Geometry check sheet. Reference: the model listing, model coordinates, mm. Face numbers are marked on the shaded views. A direction names the side the tool comes from. Coordinates: 2 decimals unless noted, no trailing zeros. Loops run counter-clockwise (first coordinate to the right, second up) from the corner with the lowest first, then second, coordinate; pieces in that order, holes last. Notation, with made-up numbers: M 73.5,6 L 131.5,6 A17 ccw 131.5,21 Z; hole C 23,25.5 d5. An arc over 180 degrees is marked long. One line per question, with ' | ' between items. Start each with the question number.
from build123d import *

# Parameters (mm, degrees)
SKETCH1_W                      = 100
SKETCH1_H                      = 59
BOSS_EXTRUDE1_DEPTH            = 12
SKETCH2_W                      = 92
SKETCH2_H                      = 54
CUT_EXTRUDE1_DEPTH             = 60.281109976
SKETCH3_W                      = 54
SKETCH3_H                      = 2.75
CUT_EXTRUDE2_DEPTH             = 1.25
SKETCH4_W                      = 54
SKETCH4_H                      = 2.75
CUT_EXTRUDE3_DEPTH             = 1.25
SKETCH5_W                      = 92
SKETCH5_H                      = 2.75
CUT_EXTRUDE4_DEPTH             = 1.25
SKETCH6_W                      = 92
SKETCH6_H                      = 2.75
CUT_EXTRUDE5_DEPTH             = 1.25
FILLET1_R                      = 1
SKETCH7_W                      = 4
SKETCH7_H                      = 10
BOSS_EXTRUDE2_DEPTH            = 5
CUT_EXTRUDE6_REACH             = 103.145
SKETCH8_W                      = 8
SKETCH8_H                      = 3
CUT_EXTRUDE6_DIRECTION_2_REACH = 103.145
FILLET2_R                      = 6.35
SKETCH9_W                      = 5
SKETCH9_H                      = 2.5
BOSS_EXTRUDE3_DEPTH            = 5
SKETCH10_W                     = 5
SKETCH10_H                     = 2.5
BOSS_EXTRUDE4_DEPTH            = 5
SKETCH11_W                     = 5
SKETCH11_H                     = 2.5
BOSS_EXTRUDE5_DEPTH            = 5
SKETCH12_W                     = 5
SKETCH12_H                     = 2.5
BOSS_EXTRUDE6_DEPTH            = 4


with BuildPart() as part:
    # Sketch1 → Boss-Extrude1 (new body)
    with BuildSketch(Plane(origin=(0, 0, 0), x_dir=(1, 0, 0), z_dir=(0, 1, 0))):
        Rectangle(SKETCH1_W, SKETCH1_H)
    extrude(amount=BOSS_EXTRUDE1_DEPTH)

    # Sketch2 → Cut-Extrude1 (cut, through all)
    with BuildSketch(Plane(origin=(0, 12, 0), x_dir=(1, 0, 0), z_dir=(0, 1, 0))):
        Rectangle(SKETCH2_W, SKETCH2_H)
    extrude(amount=-CUT_EXTRUDE1_DEPTH, mode=Mode.SUBTRACT)

    # Sketch3 → Cut-Extrude2 (cut)
    with BuildSketch(Plane(origin=(-46, 0, 0), x_dir=(0, 0, -1), z_dir=(1, 0, 0))):
        with Locations((0, 3.875)):
            Rectangle(SKETCH3_W, SKETCH3_H)
    extrude(amount=-CUT_EXTRUDE2_DEPTH, mode=Mode.SUBTRACT)

    # Sketch4 → Cut-Extrude3 (cut)
    with BuildSketch(Plane.ZY.offset(-46)):
        with Locations((0, 3.875)):
            Rectangle(SKETCH4_W, SKETCH4_H)
    extrude(amount=-CUT_EXTRUDE3_DEPTH, mode=Mode.SUBTRACT)

    # Sketch5 → Cut-Extrude4 (cut)
    with BuildSketch(Plane.XY.offset(-27)):
        with Locations((0, 3.875)):
            Rectangle(SKETCH5_W, SKETCH5_H)
    extrude(amount=-CUT_EXTRUDE4_DEPTH, mode=Mode.SUBTRACT)

    # Sketch6 → Cut-Extrude5 (cut)
    with BuildSketch(Plane(origin=(0, 0, 27), x_dir=(-1, 0, 0), z_dir=(0, 0, -1))):
        with Locations((0, 3.875)):
            Rectangle(SKETCH6_W, SKETCH6_H)
    extrude(amount=-CUT_EXTRUDE5_DEPTH, mode=Mode.SUBTRACT)

    # Fillet1
    fillet1_edges = [part.edges().sort_by_distance(p)[0] for p in [
        (0, 5.25, -28.25),
        (0, 5.25, 28.25),
    ]]
    fillet(fillet1_edges, radius=FILLET1_R)

    # Sketch7 → Boss-Extrude2 (add)
    with BuildSketch(Plane.XZ):
        with Locations((-48, 0)):
            Rectangle(SKETCH7_W, SKETCH7_H)
    boss_extrude2 = extrude(amount=BOSS_EXTRUDE2_DEPTH)

    # Mirror2: Boss-Extrude2 across plane
    add(boss_extrude2.mirror(Plane(origin=(0, 0, 0), x_dir=(0, 0, 1), z_dir=(1, 0, 0))))

    # Cut-Extrude6: up to this face of the body (flat: up to its plane)
    cut_extrude6_end = Plane(part.part.faces().sort_by_distance((-47.25, 3.875, 0))[0])
    # Sketch8 → Cut-Extrude6 (cut, up to the picked face)
    with BuildSketch(Plane(origin=(-46, 0, 0), x_dir=(0, 0, -1), z_dir=(1, 0, 0)), mode=Mode.PRIVATE) as cut_extrude6_sk1:
        with Locations((0, 1)):
            Rectangle(SKETCH8_W, SKETCH8_H)
    cut_extrude6_tool1 = split(extrude(cut_extrude6_sk1.sketch, amount=-CUT_EXTRUDE6_REACH, mode=Mode.PRIVATE), bisect_by=cut_extrude6_end, keep=Keep.BOTH, mode=Mode.PRIVATE)
    add(cut_extrude6_tool1.solids().sort_by(Axis((-46, 1, 0), (-1, 0, 0)))[0], mode=Mode.SUBTRACT)

    # Cut-Extrude6 direction 2: up to this face of the body (flat: up to its plane)
    cut_extrude6_direction_2_end = Plane(part.part.faces().sort_by_distance((47.25, 3.875, 0))[0])
    # Sketch8 → Cut-Extrude6 direction 2 (cut, up to the picked face)
    with BuildSketch(Plane(origin=(-46, 0, 0), x_dir=(0, 0, -1), z_dir=(1, 0, 0)), mode=Mode.PRIVATE) as cut_extrude6_direction_2_sk1:
        with Locations((0, 1)):
            Rectangle(SKETCH8_W, SKETCH8_H)
    cut_extrude6_direction_2_tool1 = split(extrude(cut_extrude6_direction_2_sk1.sketch, amount=CUT_EXTRUDE6_DIRECTION_2_REACH, mode=Mode.PRIVATE), bisect_by=cut_extrude6_direction_2_end, keep=Keep.BOTH, mode=Mode.PRIVATE)
    add(cut_extrude6_direction_2_tool1.solids().sort_by(Axis((-46, 1, 0), (1, 0, 0)))[0], mode=Mode.SUBTRACT)

    # Fillet2
    # the kernel refuses this fillet: 6.35 mm, written as the material it adds along each edge
    with BuildSketch(Plane(origin=(-46, 18.375, -27), x_dir=(1, 0, 0), z_dir=(0, -1, 0))) as fillet2_piece_1_section:
        with BuildLine():
            CenterArc((FILLET2_R, FILLET2_R), FILLET2_R, 180, 90)
            Line((0, FILLET2_R), (0, 0))
            Line((0, 0), (FILLET2_R, 0))
        make_face()
    fillet2_piece_1 = extrude(amount=18.375, mode=Mode.PRIVATE)
    fillet2_piece_1 = split(fillet2_piece_1, bisect_by=Plane(origin=(-44.562391024, 5.25, -25.562391024), z_dir=(0, 1, 0)), keep=Keep.TOP, mode=Mode.PRIVATE)
    fillet2_piece_1 = split(fillet2_piece_1, bisect_by=Plane(origin=(-44.562391024, 12, -25.562391024), z_dir=(0, -1, 0)), keep=Keep.TOP, mode=Mode.PRIVATE)
    add(fillet2_piece_1)
    with BuildSketch(Plane(origin=(-46, 2.5, -27), x_dir=(1, 0, 0), z_dir=(0, -1, 0)), Plane(origin=(-46, 2.5, 27), x_dir=(0, 0, -1), z_dir=(0, -1, 0))) as fillet2_piece_2:
        with BuildLine():
            CenterArc((FILLET2_R, FILLET2_R), FILLET2_R, 180, 90)
            Line((0, FILLET2_R), (0, 0))
            Line((0, 0), (FILLET2_R, 0))
        make_face()
    extrude(amount=2.5)
    with BuildSketch(Plane(origin=(46, 18.375, -27), x_dir=(-1, 0, 0), z_dir=(0, -1, 0))) as fillet2_piece_3_section:
        with BuildLine():
            CenterArc((FILLET2_R, -FILLET2_R), FILLET2_R, 90, 90)
            Line((0, -FILLET2_R), (0, 0))
            Line((0, 0), (FILLET2_R, 0))
        make_face()
    fillet2_piece_3 = extrude(amount=18.375, mode=Mode.PRIVATE)
    fillet2_piece_3 = split(fillet2_piece_3, bisect_by=Plane(origin=(44.562391024, 5.25, -25.562391024), z_dir=(0, 1, 0)), keep=Keep.TOP, mode=Mode.PRIVATE)
    fillet2_piece_3 = split(fillet2_piece_3, bisect_by=Plane(origin=(44.562391024, 12, -25.562391024), z_dir=(0, -1, 0)), keep=Keep.TOP, mode=Mode.PRIVATE)
    add(fillet2_piece_3)
    with BuildSketch(Plane(origin=(46, 2.5, -27), x_dir=(-1, 0, 0), z_dir=(0, -1, 0)), Plane(origin=(46, 2.5, 27), x_dir=(0, 0, -1), z_dir=(0, -1, 0))) as fillet2_piece_4:
        with BuildLine():
            CenterArc((FILLET2_R, -FILLET2_R), FILLET2_R, 90, 90)
            Line((0, -FILLET2_R), (0, 0))
            Line((0, 0), (FILLET2_R, 0))
        make_face()
    extrude(amount=2.5)
    with BuildSketch(Plane(origin=(-46, 18.375, 27), x_dir=(0, 0, -1), z_dir=(0, -1, 0))) as fillet2_piece_5_section:
        with BuildLine():
            CenterArc((FILLET2_R, FILLET2_R), FILLET2_R, 180, 90)
            Line((0, FILLET2_R), (0, 0))
            Line((0, 0), (FILLET2_R, 0))
        make_face()
    fillet2_piece_5 = extrude(amount=18.375, mode=Mode.PRIVATE)
    fillet2_piece_5 = split(fillet2_piece_5, bisect_by=Plane(origin=(-44.562391024, 12, 25.562391024), z_dir=(0, -1, 0)), keep=Keep.TOP, mode=Mode.PRIVATE)
    fillet2_piece_5 = split(fillet2_piece_5, bisect_by=Plane(origin=(-44.562391024, 5.25, 25.562391024), z_dir=(0, 1, 0)), keep=Keep.TOP, mode=Mode.PRIVATE)
    add(fillet2_piece_5)
    with BuildSketch(Plane(origin=(46, 18.375, 27), x_dir=(0, 0, -1), z_dir=(0, -1, 0))) as fillet2_piece_6_section:
        with BuildLine():
            CenterArc((FILLET2_R, -FILLET2_R), FILLET2_R, 90, 90)
            Line((0, -FILLET2_R), (0, 0))
            Line((0, 0), (FILLET2_R, 0))
        make_face()
    fillet2_piece_6 = extrude(amount=18.375, mode=Mode.PRIVATE)
    fillet2_piece_6 = split(fillet2_piece_6, bisect_by=Plane(origin=(44.562391024, 12, 25.562391024), z_dir=(0, -1, 0)), keep=Keep.TOP, mode=Mode.PRIVATE)
    fillet2_piece_6 = split(fillet2_piece_6, bisect_by=Plane(origin=(44.562391024, 5.25, 25.562391024), z_dir=(0, 1, 0)), keep=Keep.TOP, mode=Mode.PRIVATE)
    add(fillet2_piece_6)
    # the kernel refuses this fillet: 6.35 mm, written as the material it takes off along each edge
    with BuildSketch(Plane(origin=(-50, -15.875, -29.5), x_dir=(1, 0, 0), z_dir=(0, 1, 0)), Plane(origin=(-50, -15.875, 29.5), x_dir=(0, 0, -1), z_dir=(0, 1, 0))) as fillet2_2_piece_1:
        with BuildLine():
            CenterArc((FILLET2_R, -FILLET2_R), FILLET2_R, 90, 90)
            Line((0, -FILLET2_R), (0, 0))
            Line((0, 0), (FILLET2_R, 0))
        make_face()
    extrude(amount=43.75, mode=Mode.SUBTRACT)
    with BuildSketch(Plane(origin=(50, -15.875, 29.5), x_dir=(0, 0, -1), z_dir=(0, 1, 0)), Plane(origin=(50, -15.875, -29.5), x_dir=(-1, 0, 0), z_dir=(0, 1, 0))) as fillet2_2_piece_2:
        with BuildLine():
            CenterArc((FILLET2_R, FILLET2_R), FILLET2_R, 180, 90)
            Line((0, FILLET2_R), (0, 0))
            Line((0, 0), (FILLET2_R, 0))
        make_face()
    extrude(amount=43.75, mode=Mode.SUBTRACT)

    # Sketch9 → Boss-Extrude3 (add)
    with BuildSketch(Plane(origin=(0, 0, 27), x_dir=(-1, 0, 0), z_dir=(0, 0, -1))):
        with Locations((0, 7.5)):
            Rectangle(SKETCH9_W, SKETCH9_H)
    extrude(amount=BOSS_EXTRUDE3_DEPTH)

    # Sketch10 → Boss-Extrude4 (add)
    with BuildSketch(Plane.XY.offset(-27)):
        with Locations((0, 7.5)):
            Rectangle(SKETCH10_W, SKETCH10_H)
    extrude(amount=BOSS_EXTRUDE4_DEPTH)

    # Sketch11 → Boss-Extrude5 (add)
    with BuildSketch(Plane.ZY.offset(-46)):
        with Locations((0, 7.5)):
            Rectangle(SKETCH11_W, SKETCH11_H)
    extrude(amount=BOSS_EXTRUDE5_DEPTH)

    # Sketch12 → Boss-Extrude6 (add)
    with BuildSketch(Plane(origin=(-46, 0, 0), x_dir=(0, 0, -1), z_dir=(1, 0, 0))):
        with Locations((0, 7.5)):
            Rectangle(SKETCH12_W, SKETCH12_H)
    extrude(amount=BOSS_EXTRUDE6_DEPTH)


solid = part.part
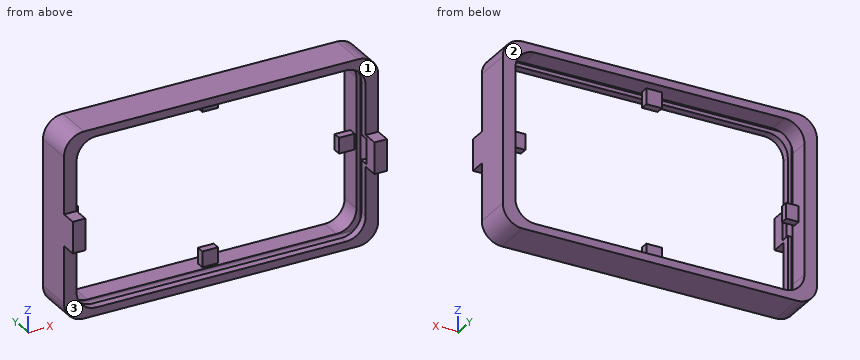
1. Sectioned sample at C-C (z = 13.5). Record the cut outline in (x, y).
2. Depth check by flat-ended pin: pin 1 Ø0.6 at (y, z) = (4, -27.5) entering from -X; pin 2 Ø1.4 at (y, z) = (4.5, 27.5) entering from -X; pin 3 Ø2 at (y, z) = (7.5, 24.5) entering from +X. Enter the tip coordinate at first touch or a pass-through.
3. Thickness scan on line 1 (X direction, y = 3.25, z = -12.5); line 2 (X direction, y = 7.5, z = -18.5); line 3 (Z direction, x = -17.5, y = 4.25). Record the ranges inside material, lowest first.
4. Tool access check on the marked faces 1, 2 and 3. Record the directions out of +Z, -Z, +X, -X, +Y, -Y that give a thin tool (end or side, any length) a straight path to the whole face; none if there is none.
5. Sectioned sample at A-A (x = -32). Record the cut outline in (y, z), and give its area (3 significant figures).
6. Sectioned sample at D-D (y = -3). Record the cut outline in (x, z).
Result:
1) outline: M -50,0 L -46,0 L -46,2.5 L -47.25,2.5 L -47.25,5.25 L -46,5.25 L -46,12 L -50,12 Z; M 46,0 L 50,0 L 50,12 L 46,12 L 46,5.25 L 47.25,5.25 L 47.25,2.5 L 46,2.5 Z
2) pin 1: stops at x = -48.54 | pin 2: stops at x = -48.85 | pin 3: stops at x = 49.99
3) line 1: x = -50 to -47.25, 47.25 to 50 | line 2: x = -50 to -46, 46 to 50 | line 3: z = -29.5 to -28.25, 28.25 to 29.5
4) face 1: +Z, +X, -X, -Y | face 2: +Z, -Z, +X, -X, +Y | face 3: -Z, +X, -X, -Y
5) outline: M 0,-29.5 L 12,-29.5 L 12,-27 L 5.25,-27 L 5.25,-27.25 A1 cw 4.25,-28.25 L 2.5,-28.25 L 2.5,-27 L 0,-27 Z; M 0,27 L 2.5,27 L 2.5,28.25 L 4.25,28.25 A1 cw 5.25,27.25 L 5.25,27 L 12,27 L 12,29.5 L 0,29.5 Z | area: 53.6 mm2
6) outline: M -50,-5 L -46,-5 L -46,5 L -50,5 Z; M 46,-5 L 50,-5 L 50,5 L 46,5 Z
